```python
from build123d import *

# Parameters (mm, degrees)
FILLET1_R          = 0.635
CUT_EXTRUDE1_DEPTH = 2.4
FILLET2_R          = 0.635


with BuildPart() as part:
    # Sketch2 → Revolve1 (revolve)
    with BuildSketch(Plane.XY):
        Polygon((0, 4.65), (4.875, 4.65), (4.875, 2.65), (2.5, 2.65), (2.413, 0.35), (2.413, -4.65), (0, -4.65), align=None)
    revolve(axis=Axis((0, -4.65, 0), (0, 1, 0)))

    # Fillet1
    fillet1_edges = [part.edges().sort_by_distance(p)[0] for p in [
        (-2.5, 2.65, 0),
        (-4.875, 2.65, 0),
        (-4.875, 4.65, 0),
    ]]
    fillet(fillet1_edges, radius=FILLET1_R)

    # Sketch3 → Cut-Extrude1 (cut)
    with BuildSketch(Plane(origin=(0, 4.65, 0), x_dir=(1, 0, 0), z_dir=(0, 1, 0))):
        Polygon((0, 1.732050808), (-1.5, 0.866025404), (-1.5, -0.866025404), (0, -1.732050808), (1.5, -0.866025404), (1.5, 0.866025404), align=None)
    extrude(amount=-CUT_EXTRUDE1_DEPTH, mode=Mode.SUBTRACT)

    # Fillet2
    fillet2_edges = [part.edges().sort_by_distance(p)[0] for p in [
        (0.75, 4.65, -1.299038106),
        (-0.75, 4.65, -1.299038106),
        (-1.5, 4.65, 0),
        (-0.75, 4.65, 1.299038106),
        (0.75, 4.65, 1.299038106),
        (1.5, 4.65, 0),
    ]]
    fillet(fillet2_edges, radius=FILLET2_R)


solid = part.part
```
Input: part model. Units: mm. Frame: model coordinates. A direction names the side the tool comes from. Round coordinates to 2 decimals unless told otherwise and drop trailing zeros. Loops run counter-clockwise (first coordinate to the right, second up) from the corner with the lowest first, then second, coordinate; pieces in that order, holes last. Notation, with made-up numbers: (-1.5, -32) -> (44.5, -32) arc R30 ccw to (44.5, -9) -> close; hole circle Ø2 at (56.5, 51.25). An arc over 180 degrees is marked (long way). Use one line per item in the form item = value. Start each with the question number.
Item 1: Material intervals for L1, parallel to Y at x = 1, z = -0.5; L2, parallel to X at y = 2, z = 0; L3, parallel to Z at x = 0.5, y = 3.75, sorted ascending. Write a range as from..to.
Item 2: Contact query for flat-ended pins moving along their axis: pin 1 Ø1 at (x, y) = (-0.5, -1) entering from -Z; pin 2 Ø2 at (x, y) = (3.5, 3) entering from +Z; pin 3 Ø1.5 at (x, y) = (1, 1) entering from +Z. Output: stop coordinate, or through.
Item 3: Section query A-A on y = 3.5. Return the cut outline in (x, z) (3 decimals).
Item 4: Mould query, pull axis X, two halves, no side actions, for faces 4 (the face through (0, -4.65, 0)), 5 (the face through (-0.53, 1.183, 2.386)), 6 (the face through (-0.86, 4.47, -1.46)). Classes: pulls with the +X half, pulls with the -X half, needs draft (parallel to the pull), parting line crosses it, or undercut.
Item 5: Section query B-B on z = 0. Return the cut outline in (x, y) (3 decimals).
Item 6: Set-up query: faces 1 (the face through (1.5, 3, 0)), 2 (the face through (-0.635, 3.645, -4.834)), 3 (the face through (-1.915, -2.185, 1.468)). Return all of +Z, -Z, +X, -X, +Y, -Y with unobstructed straight access to the full face (end or side cutting, diameter ignored); none if empty.
Item 7: Section query C-C on y = -1. Return the cut outline in (x, z).
Ans:
q1.L1 = -4.65..2.25
q1.L2 = -2.48..2.48
q1.L3 = -4.85..-1.44, 1.44..4.85
q2.pin_1 = -2.41
q2.pin_2 = 4.17
q2.pin_3 = 2.43
q3.outline = circle Ø9.75 at (0, 0); hole (-1.5, -0.866) -> (0, -1.732) -> (1.5, -0.866) -> (1.5, 0.866) -> (0, 1.732) -> (-1.5, 0.866) -> close
q4.face_4 = needs draft
q4.face_5 = parting line crosses it
q4.face_6 = undercut
q5.outline = (-4.875, 3.285) arc R0.635 ccw to (-4.24, 2.65) -> (-3.111, 2.65) arc R0.635 cw to (-2.477, 2.039) -> (-2.413, 0.35) -> (-2.413, -4.65) -> (2.413, -4.65) -> (2.413, 0.35) -> (2.477, 2.039) arc R0.635 cw to (3.111, 2.65) -> (4.24, 2.65) arc R0.635 ccw to (4.875, 3.285) -> (4.875, 4.015) arc R0.635 ccw to (4.24, 4.65) -> (2.135, 4.65) arc R0.635 ccw to (1.5, 4.015) -> (1.5, 2.25) -> (-1.5, 2.25) -> (-1.5, 4.015) arc R0.635 ccw to (-2.135, 4.65) -> (-4.24, 4.65) arc R0.635 ccw to (-4.875, 4.015) -> close
q6.face_1 = +Y
q6.face_2 = +Y, -Y
q6.face_3 = -Y
q7.outline = circle Ø4.83 at (0, 0)
